CAD build for the part. Positions are in the model's coordinates, mm. Give positions to 0.01 mm unless a question says otherwise; leave off trailing zeros. Order: outer loops, then holes, each group sorted by start corner. A loop starts at its lowest first (then second) coordinate and runs counter-clockwise, first axis right, second up.
from build123d import *

# Parameters (mm, degrees)
SKETCH1_R           = 3
SKETCH1_R_2         = 1.688307965
BOSS_EXTRUDE1_DEPTH = 4
FILLET1_R           = 4
FILLET4_R           = 30
FILLET5_R           = 40
FILLET6_R           = 5
SKETCH6_R           = 3
CUT_EXTRUDE2_DEPTH  = 34


with BuildPart() as part:
    # Sketch1 → Boss-Extrude1 (new body)
    with BuildSketch(Plane.XY):
        Polygon((7.903848118, 3.731035494), (-21.954412971, -29.93622226), (-30.932348372, -21.974019303), (-3.972092158, 8.4255372), (-3.133542372, 39.046414738), (8.861960559, 38.717919044), align=None)
        with Locations((-21.135245367, -19.969830514)):
            Circle(SKETCH1_R, mode=Mode.SUBTRACT)
        with Locations((2.645211964, 30.885164937)):
            Circle(SKETCH1_R_2, mode=Mode.SUBTRACT)
    extrude(amount=BOSS_EXTRUDE1_DEPTH)

    # Fillet1
    fillet1_edges = [part.edges().sort_by_distance(p)[0] for p in [
        (-30.932348372, -21.974019303, 2),
        (-21.954412971, -29.93622226, 2),
    ]]
    fillet(fillet1_edges, radius=FILLET1_R)

    # Fillet4
    fillet4_edges = [part.edges().sort_by_distance(p)[0] for p in [
        (7.903848118, 3.731035494, 2),
    ]]
    fillet(fillet4_edges, radius=FILLET4_R)

    # Fillet5
    fillet5_edges = [part.edges().sort_by_distance(p)[0] for p in [
        (-3.972092158, 8.4255372, 2),
    ]]
    fillet(fillet5_edges, radius=FILLET5_R)

    # Fillet6
    fillet6_edges = [part.edges().sort_by_distance(p)[0] for p in [
        (-3.133542372, 39.046414738, 2),
        (8.861960559, 38.717919044, 2),
    ]]
    fillet(fillet6_edges, radius=FILLET6_R)

    # Sketch6 → Cut-Extrude2 (cut)
    with BuildSketch(Plane.XY.offset(4)):
        with Locations((-0.123058619, 6.904032873)):
            Circle(SKETCH6_R)
    extrude(amount=-CUT_EXTRUDE2_DEPTH, mode=Mode.SUBTRACT)


solid = part.part
1. Wall check: line 1 (Y direction, x = 2, z = 2.65) (3 decimals); line 2 (Y direction, x = 1.5, z = 2.15); line 3 (Y direction, x = 4, z = 2.8). Give the ranges that are in metal, low to high.
2. Pin check, flat tips, straight feed: P1, Ø1, axis at x = -24.5, z = 3.5, coming from the -Y side; P2, Ø1, axis at x = -12, z = 2.5, coming from the +Y side. Stop position of each tip, or through.
3. Saw through at A-A on x = -20.5. Give the cut face in (y, z), plus the area to 3 significant figures.
4. Saw through at B-B on z = 1.75. Give the cut face in (x, y), plus the area to 3 significant figures.
5. Mould opens along X. For faces 1 (the flat face through (-6, 5, 0)), 2 (the flat face through (-21.06, -10.84, 1.97)), 3 (the cylindrical face through (2.279, 29.237, 1.972)) say: released by +X, released by -X, zero draft, split by the parting line, or undercut.
6. Saw through at C-C on x = -2.5. Give the cut face in (y, z).
7. Saw through at D-D on y = 11. Give the cut face in (x, z).
Reported:
1. line 1: y = -2.815 to 4.784, 9.024 to 29.325, 32.445 to 38.906
1. line 2: y = -3.45 to 4.38, 9.43 to 29.64, 32.13 to 38.91
1. line 3: y = 0.13 to 29.88, 31.89 to 38.85
2. P1: stops at y = -27.91
2. P2: stops at y = 0.15
3. outline: (-27.87, 0) - (-22.9, 0) - (-22.9, 4) - (-27.87, 4) - close; (-17.04, 0) - (-10.21, 0) - (-10.21, 4) - (-17.04, 4) - close
3. area: 47.2 mm2
4. outline: (-28.28, -18.98) arc R4 ccw to (-27.94, -24.63) - (-24.95, -27.28) arc R4 ccw to (-19.3, -26.94) - (0.66, -4.44) arc R30 ccw to (8.2, 14.65) - (8.73, 33.72) arc R5 ccw to (3.86, 38.85) - (1.86, 38.91) arc R5 ccw to (-3.27, 34.05) - (-3.57, 22.98) arc R40 cw to (-13.63, -2.47) - close; hole circle Ø6 at (-21.14, -19.97); hole circle Ø6 at (-0.12, 6.9); hole circle Ø3.38 at (2.65, 30.89)
4. area: 835 mm2
5. face 1: zero draft
5. face 2: released by -X
5. face 3: undercut
6. outline: (-8, 0) - (5.07, 0) - (5.07, 4) - (-8, 4) - close; (8.73, 0) - (36.58, 0) - (36.58, 4) - (8.73, 4) - close
7. outline: (-5.76, 0) - (7.88, 0) - (7.88, 4) - (-5.76, 4) - close
